Design review of the part built by this model. Coordinates are the model's own, in mm. Give positions to 0.01 mm unless a question says otherwise; leave off trailing zeros. Write each loop counter-clockwise with the first axis right and the second up, starting at its lowest first coordinate (ties: lowest second). Pieces come first, ordered by that corner, then holes. Notation, with made-up numbers: M 74,-0.5 L 99,-0.5 A9 cw 99,9.5 Z; hole C 36,-12 d3. An arc over 180 degrees is marked long. Use a Markdown table: item, result. Add a question column.
```python
from build123d import *


# Not quite as in the source:
# - a feature of the source that left no trace in its solid (it failed there, or was rolled back) is left out
# - a feature names something its author has since deleted; it is built from what else it names


with BuildPart() as f1:
    # F0 (on Front) → F1 (revolve)
    with BuildSketch(Plane.XZ):
        with BuildLine():
            Line((8.2452101406, -109.7828151841), (4.4973873494, 0.1533200233))
            ThreePointArc((4.4973873494, 0.1533200233), (3.1273039423, 3.2357333098), (0, 4.5))
            Line((0, 4.5), (0, 2.8))
            ThreePointArc((0, 2.8), (1.9458780086, 2.0133451706), (2.7983743507, 0.0953991256))
            Line((2.7983743507, 0.0953991256), (6.4590447751, -107.2842666566))
            Line((6.4590447751, -107.2842666566), (6.4726732216, -107.684034421))
            Line((6.4726732216, -107.684034421), (6.4863016682, -108.0838021854))
            Line((6.4863016682, -108.0838021854), (6.5033471227, -108.5838021854))
            Line((6.5033471227, -108.5838021854), (6.5442225658, -109.7828151841))
            Line((6.5442225658, -109.7828151841), (8.2452101406, -109.7828151841))
        make_face()
        with BuildLine():
            Line((6.4726732216, -107.684034421), (6.4590447751, -107.2842666566))
            ThreePointArc((6.4590447751, -107.2842666566), (6.2505990382, -107.4374019066), (6.1726732216, -107.684034421))
            Line((6.1726732216, -107.684034421), (6.4726732216, -107.684034421))
        make_face()
        with BuildLine():
            ThreePointArc((6.1726732216, -107.684034421), (6.2615032541, -107.9372537095), (6.4863016682, -108.0838021854))
            Line((6.4863016682, -108.0838021854), (6.4726732216, -107.684034421))
            Line((6.4726732216, -107.684034421), (6.1726732216, -107.684034421))
        make_face()
    revolve(axis=Axis((0, 0, -52.7819509467), (0, 0, 1)))


solid = f1.part
```
(1) The part is to be moulded in two halves that separate along X. For faces 1 (the conical face through (-0.83, 6.29, -54.05)), 2 (the conical face through (4.44, 1.4, -54.35)), 3 (the flat face through (6, 4, -109.783)), say which applies: released by +X, released by -X, zero draft, split by the parting line, or undercut.
(2) For pin 1 (1.5 mm diameter, centred on y = 4, z = -8, fed in from +X); pin 2 (2 mm diameter, centred on y = 6.5, z = -95, fed in from -X); pin 3 (1 mm diameter, centred on x = -2, z = -68.5, fed in from -Y), all flat-tipped, find the tip position at first contact; note any pin that passes through.
(3) Add section A-A on z = -9.5. Give the boundary of the cut face in (x, y), then the cut area to 3 significant figures.
(4) Add section B-B on z = -44.5. Give the boundary of the cut face in (x, y).
(5) Wall thickness on L1, parallel to Y at x = 1.5, z = -81; L2, parallel to X at y = -2.25, z = -2; L3, parallel to Y at x = -0.5, z = -19: over which ranges is each line inside the solid? List them lowest first.
From the geometry:
| question | item | result |
|---|---|---|
| 1 | face 1 | split by the parting line |
| 1 | face 2 | undercut |
| 1 | face 3 | zero draft |
| 2 | pin 1 | stops at x = 3.5 |
| 2 | pin 2 | stops at x = -5.45 |
| 2 | pin 3 | stops at y = -6.67 |
| 3 | outline | C 0,0 d9.65; hole C 0,0 d6.25 |
| 3 | area | 42.5 mm^2 |
| 4 | outline | C 0,0 d12.04; hole C 0,0 d8.64 |
| 5 | L1 | y = -7.11 to -5.36, 5.36 to 7.11 |
| 5 | L2 | x = -3.98 to -1.78, 1.78 to 3.98 |
| 5 | L3 | y = -5.13 to -3.41, 3.41 to 5.13 |
